Can you work these out from the model? Positions are in its coordinate system, mm. A direction names the side the tool comes from. Coordinates: 2 decimals unless noted, no trailing zeros. Loops run counter-clockwise (first coordinate to the right, second up) from the corner with the lowest first, then second, coordinate; pieces in that order, holes last.
```python
from build123d import *

# Parameters (mm, degrees)
F2_R      = 2
F2_R_2    = 1.75
F3_DEPTH  = 2
F1_R      = 4
F1_R_2    = 3.4
F4_DEPTH  = 2
F7_DEPTH  = 1.9
F8_DEPTH  = 1.9
F9_DEPTH  = 0.9
F10_DEPTH = 1.9


with BuildPart() as f3:
    # F2 (on offset) → F3 (new body)
    with BuildSketch(Plane.XZ.offset(10)):
        Circle(F2_R)
        Circle(F2_R_2, mode=Mode.SUBTRACT)
    extrude(amount=F3_DEPTH)



with BuildPart() as f4:
    # F1 (on Front) → F4 (new body)
    with BuildSketch(Plane.XZ):
        Circle(F1_R)
        Circle(F1_R_2, mode=Mode.SUBTRACT)
    extrude(amount=-F4_DEPTH)


with BuildPart() as f3_1:
    add(f3.part)

    add(f4.part)  # F6 merges F4
    # F5 (on Right) → F6 (revolve)
    with BuildSketch(Plane.YZ):
        Polygon((-10, -2), (0, -4), (0, -3.4), (-10, -1.75), align=None)
    revolve(axis=Axis((0, -5, 0), (0, -1, 0)))

    # F7 (cut): a face of the model
    f7_faces = [f3_1.faces().sort_by_distance(p)[0] for p in [
        (-1.9434314575, -12, 0),
    ]]
    extrude(f7_faces, amount=-F7_DEPTH, mode=Mode.SUBTRACT)

    # F8 (cut): a face of the model
    f8_faces = [f3_1.faces().sort_by_distance(p)[0] for p in [
        (-3.886862915, 2, 0),
    ]]
    extrude(f8_faces, amount=-F8_DEPTH, mode=Mode.SUBTRACT)

    # F9 (add): a face of the model
    f9_faces = [f3_1.faces().sort_by_distance(p)[0] for p in [
        (-1.9434314575, -10.1, 0),
    ]]
    extrude(f9_faces, amount=F9_DEPTH)

    # F10 (add): a face of the model
    f10_faces = [f3_1.faces().sort_by_distance(p)[0] for p in [
        (-3.886862915, 0.1, 0),
    ]]
    extrude(f10_faces, amount=F10_DEPTH)


solid = f3_1.part
```
Item 1: On a 3-axis mill with a long thin cutter (end or side, diameter ignored), from which of +Z, -Z, +X, -X, +Y, -Y can I reach the whole of each face in a straight line? I mean faces 1 (the face through (-0.434, -10.493, -1.952)), 2 (the face through (-1.56, -5.07, 2.034)). Say none if no direction works.
Results are:
face 1: -Y
face 2: +Y
Item 2: Suppose I cut it at B-B, the plane z = 0. Please give me the cut outline in (x, y), plus the area to 3 significant figures.
Results are:
outline: (-4, 0) - (-2, -10) - (-2, -11) - (-1.75, -11) - (-1.75, -10) - (-3.4, 0) - (-3.4, 2) - (-4, 2) - close; (1.75, -11) - (2, -11) - (2, -10) - (4, 0) - (4, 2) - (3.4, 2) - (3.4, 0) - (1.75, -10) - close
area: 11.4 mm2
Item 3: Suppose I cut it at C-C, the plane y = -1.5. Please give me the cut outline in (x, z) (1 decimal), plus the area to 3 significant figures.
Results are:
outline: circle Ø7.4 at (0, 0); hole circle Ø6.3 at (0, 0)
area: 11.8 mm2
Item 4: Suppose I cut it at D-D, the plane y = 0.5. Please give me the cut outline in (x, z).
Results are:
outline: circle Ø8 at (0, 0); hole circle Ø6.8 at (0, 0)
Item 5: We'd pull the mould along X, two halves only. Please class faces 3 (the face through (-0.867, 0.986, -3.905)), 4 (the face through (-0.74, 0.99, -3.32)), 5 (the face through (1.617, -10.493, -0.67)), 6 (the face through (-2, 2, -3)): +X half, -X half, draft (parallel to the pull), parting line (faces both ways), or undercut.
Results are:
face 3: parting line
face 4: undercut
face 5: undercut
face 6: draft
Item 6: I need wall thicknesses on line 1 along Z through (x, y) = (0, 0.55); line 2 along Z through (x, y) = (0, -10.75). Which ranges of each line are inside material? Lowest first, please.
Results are:
line 1: z = -4 to -3.4, 3.4 to 4
line 2: z = -2 to -1.75, 1.75 to 2
Item 7: I'm going to push flat-ended pins straight in: P1, Ø3, axis at y = -2, z = 1, coming from the +X side; P2, Ø3, axis at x = 0, z = 0, coming from the -Y side; P3, Ø3, axis at y = -4, z = 3, coming from the -X side. Where does each tip first touch, or does it pass through?
Results are:
P1: stops at x = 3.85
P2: passes through
P3: stops at x = -2.9
Item 8: Suppose I cut it at A-A, the plane x = 0. Please give me the cut outline in (y, z), plus the area to 3 significant figures.
Results are:
outline: (-11, -2) - (-10, -2) - (0, -4) - (2, -4) - (2, -3.4) - (0, -3.4) - (-10, -1.75) - (-11, -1.75) - close; (-11, 1.75) - (-10, 1.75) - (0, 3.4) - (2, 3.4) - (2, 4) - (0, 4) - (-10, 2) - (-11, 2) - close
area: 11.4 mm2
